Check sheet for the modelled part. Datum: model origin and axes. Units: mm. A direction names the side the tool comes from. Coordinates: 2 decimals unless noted, no trailing zeros. Loops run counter-clockwise (first coordinate to the right, second up) from the corner with the lowest first, then second, coordinate; pieces in that order, holes last. Notation, with made-up numbers: (64, 74) - (87, 74) arc R23 ccw to (87, 104) - close; hole circle Ø10 at (82, 70). An arc over 180 degrees is marked (long way). Use a Markdown table: item, result. Add a question column.
1) Sectioned sample at D-D, the plane y = -158.5. Enter the section's corners in (x, z).
2) Tool access check on faces 1 (the flat face through (-1, -130, 30)), 2 (the flat face through (-1, 130, 32)), 3 (the flat face through (1, 3, 0)), 4 (the flat face through (80, -2, 30)), 5 (the flat face through (-80, -2, 30)). Record the directions out of +Z, -Z, +X, -X, +Y, -Y that give a thin tool (end or side, any length) a straight path to the whole face; none if there is none.
3) Sectioned sample at B-B, the plane x = 29. Enter the section's corners in (y, z).
4) Thickness scan on line 1 (Z direction, x = -129.5, y = -98); line 2 (Y direction, x = 21.5, z = 26.5); line 3 (Y direction, x = 50, z = 22). Record the ranges inside material, lowest first.
5) Sectioned sample at C-C, the plane x = -100. Enter the section's corners in (y, z).
6) Sectioned sample at A-A, the plane y = -108. Enter the section's corners in (x, z), then the cut area to 3 significant figures.
7) Go/stop test with flat-tipped pins: P1, Ø8, axis at y = -57, z = 29.5, coming from the +X side; P2, Ø8, axis at y = -16.5, z = 31.5, coming from the -X side; P3, Ø7.5, axis at x = 34, z = 30.5, coming from the +Y side. Record where each tip stops, or that it passes through.
from build123d import *

# Parameters (mm, degrees)
F0_W     = 320
F0_H     = 400
F1_DEPTH = 25
F3_R     = 5
F4_W     = 160
F4_H     = 260
F5_DEPTH = 15
F6_R     = 5


with BuildPart() as f1:
    # F0 (on Top) → F1 (new body)
    with BuildSketch(Plane.XY):
        with Locations((3.315994, 0)):
            Rectangle(F0_W, F0_H)
    extrude(amount=F1_DEPTH)

    # F3
    f3_edges = [f1.edges().sort_by_distance(p)[0] for p in [
        (-156.684006, 0, 25),
        (163.315994, 0, 25),
        (3.315994, -200, 25),
    ]]
    fillet(f3_edges, radius=F3_R)

    # F4 (on face) → F5 (join)
    with BuildSketch(Plane.XY.offset(25)):
        Rectangle(F4_W, F4_H)
    extrude(amount=F5_DEPTH)

    # F6
    f6_edges = [f1.edges().sort_by_distance(p)[0] for p in [
        (-80, 0, 40),
        (0, -130, 40),
        (80, 0, 40),
    ]]
    fillet(f6_edges, radius=F6_R)


solid = f1.part
Solved:
| question | item | result |
|---|---|---|
| 1 | outline | (-156.68, 0) - (163.32, 0) - (163.32, 20) arc R5 ccw to (158.32, 25) - (-151.68, 25) arc R5 ccw to (-156.68, 20) - close |
| 2 | face 1 | +Z, +X, -X, -Y |
| 2 | face 2 | +Z, +X, -X, +Y |
| 2 | face 3 | -Z, +X, -X, +Y, -Y |
| 2 | face 4 | +Z, +X, +Y, -Y |
| 2 | face 5 | +Z, -X, +Y, -Y |
| 3 | outline | (-200, 0) - (200, 0) - (200, 25) - (130, 25) - (130, 40) - (-125, 40) arc R5 ccw to (-130, 35) - (-130, 25) - (-195, 25) arc R5 ccw to (-200, 20) - close |
| 4 | line 1 | z = 0 to 25 |
| 4 | line 2 | y = -130 to 130 |
| 4 | line 3 | y = -199.58 to 200 |
| 5 | outline | (-200, 0) - (200, 0) - (200, 25) - (-195, 25) arc R5 ccw to (-200, 20) - close |
| 6 | outline | (-156.68, 0) - (163.32, 0) - (163.32, 20) arc R5 ccw to (158.32, 25) - (80, 25) - (80, 35) arc R5 ccw to (75, 40) - (-75, 40) arc R5 ccw to (-80, 35) - (-80, 25) - (-151.68, 25) arc R5 ccw to (-156.68, 20) - close |
| 6 | area | 10,400 mm2 |
| 7 | P1 | stops at x = 80 |
| 7 | P2 | stops at x = -80 |
| 7 | P3 | stops at y = 130 |
